```python
from build123d import *

# Parameters (mm, degrees)
ESQUISSE1_W        = 32
ESQUISSE1_H        = 3
BOSS_EXTRU_2_DEPTH = 2
ESQUISSE4_R        = 1.5
BOSS_EXTRU_3_DEPTH = 6
ESQUISSE5_R        = 1.9
BOSS_EXTRU_4_DEPTH = 1
CONG_13_R          = 1.5
CONG_14_R          = 1.5
CONG_16_R          = 1.5
CONG_17_R          = 1.5


with BuildPart() as part:
    # Esquisse1 → Boss.-Extru.2 (new body)
    with BuildSketch(Plane(origin=(-13.705479482, 0.648434545, 0), x_dir=(1, 0, 0), z_dir=(0, 0, 1))):
        with Locations((47.215800187, 12.683032093)):
            Rectangle(ESQUISSE1_W, ESQUISSE1_H)
    extrude(amount=BOSS_EXTRU_2_DEPTH)

    # Esquisse4 → Boss.-Extru.3 (add)
    with BuildSketch(Plane(origin=(-13.705479482, 4.052004393, 2), x_dir=(1, 0, 0), z_dir=(0, 0, 1))):
        with Locations(Location((32.71685212, 9.269475593, 0), (0, 0, 263.384796373))):
            Circle(ESQUISSE4_R)
        with Locations(Location((61.71685212, 9.250376763, 0), (0, 0, 258.698543871))):
            Circle(ESQUISSE4_R)
    extrude(amount=BOSS_EXTRU_3_DEPTH)

    # Esquisse5 → Boss.-Extru.4 (add)
    with BuildSketch(Plane(origin=(-13.705479482, 4.052004393, 8), x_dir=(1, 0, 0), z_dir=(0, 0, 1))):
        with Locations((32.71685212, 9.269475593)):
            Circle(ESQUISSE5_R)
        with Locations((61.71685212, 9.250376763)):
            Circle(ESQUISSE5_R)
    extrude(amount=BOSS_EXTRU_4_DEPTH)

    # Congé13
    # the kernel refuses this fillet: 1.5 mm, written as the material it takes off along each edge
    with BuildSketch(Plane(origin=(49.510320705, 14.831466639, -3.75), x_dir=(0, -1, 0), z_dir=(0, 0, 1)), Plane(origin=(49.510320705, 11.831466639, -3.75), x_dir=(-1, 0, 0), z_dir=(0, 0, 1))) as cong_13_piece_1:
        with BuildLine():
            CenterArc((CONG_13_R, -CONG_13_R), CONG_13_R, 90, 90)
            Line((0, -CONG_13_R), (0, 0))
            Line((0, 0), (CONG_13_R, 0))
        make_face()
    extrude(amount=5.75, mode=Mode.SUBTRACT)

    # Congé14
    # the kernel refuses this fillet: 1.5 mm, written as the material it takes off along each edge
    with BuildSketch(Plane(origin=(17.510320705, 11.831466639, -3.75), x_dir=(0, 1, 0), z_dir=(0, 0, 1))) as cong_14_piece_1:
        with BuildLine():
            CenterArc((CONG_14_R, -CONG_14_R), CONG_14_R, 90, 90)
            Line((0, -CONG_14_R), (0, 0))
            Line((0, 0), (CONG_14_R, 0))
        make_face()
    extrude(amount=5.75, mode=Mode.SUBTRACT)
    with BuildSketch(Plane(origin=(17.510320705, 14.831466639, -3.75), x_dir=(0, -1, 0), z_dir=(0, 0, 1))) as cong_14_piece_2:
        with BuildLine():
            CenterArc((CONG_14_R, CONG_14_R), CONG_14_R, 180, 90)
            Line((0, CONG_14_R), (0, 0))
            Line((0, 0), (CONG_14_R, 0))
        make_face()
    extrude(amount=9.5, mode=Mode.SUBTRACT)

    # Congé16
    # the kernel refuses this fillet: 1.5 mm, written as the material it takes off along each edge
    with BuildSketch(Plane(origin=(48.011372638, 13.302381156, 9), x_dir=(1, 0, 0), z_dir=(0, -1, 0))) as cong_16_piece_1:
        with BuildLine():
            CenterArc((0.485786438, -1.5), CONG_16_R, 19.471220634, 70.528779366)
            Line((0.485786438, 0), (0.485786438, 0.03))
            Line((0.485786438, 0.03), (1.9, 0.03))
            Line((1.9, 0.03), (1.93, 0))
            ThreePointArc((1.93, 0), (1.93, -0.5), (1.928284271, -0.99))
            Line((1.928284271, -0.99), (1.9, -1))
        make_face()
    revolve(axis=Axis((48.011372638, 13.302381156, 9), (0, 0, 1)), mode=Mode.SUBTRACT)

    # Congé17
    # the kernel refuses this fillet: 1.5 mm, written as the material it takes off along each edge
    with BuildSketch(Plane(origin=(19.011372638, 13.321479986, 9), x_dir=(1, 0, 0), z_dir=(0, -1, 0))) as cong_17_piece_1:
        with BuildLine():
            CenterArc((0.485786438, -1.5), CONG_17_R, 19.471220634, 70.528779366)
            Line((0.485786438, 0), (0.485786438, 0.03))
            Line((0.485786438, 0.03), (1.9, 0.03))
            Line((1.9, 0.03), (1.93, 0))
            ThreePointArc((1.93, 0), (1.93, -0.5), (1.928284271, -0.99))
            Line((1.928284271, -0.99), (1.9, -1))
        make_face()
    revolve(axis=Axis((19.011372638, 13.321479986, 9), (0, 0, 1)), mode=Mode.SUBTRACT)


solid = part.part
```
Input: part model. Units: mm. Frame: model coordinates. A direction names the side the tool comes from. Coordinates: 2 decimals unless noted, no trailing zeros. Write each loop counter-clockwise with the first axis right and the second up, starting at its lowest first coordinate (ties: lowest second). Pieces come first, ordered by that corner, then holes.
1) Section B-B on x = 34. Output: boundary loops of the cut face in (y, z), and give its area (3 significant figures).
2) Pin query (flat end, axial travel): pin 1 Ø0.6 at (x, z) = (34, 0.5) entering from +Y; pin 2 Ø1 at (y, z) = (14.5, 3.5) entering from +X; pin 3 Ø1.5 at (y, z) = (12, 3.5) entering from -X; pin 4 Ø4 at (x, z) = (24.5, 8) entering from +Y. Return the tip coordinate at first contact, or that it passes through.
3) Section A-A on z = 3.75. Output: boundary loops of the cut face in (x, y), and give its area (3 significant figures).
4) Material intervals for line 1 along Z through (x, y) = (25.5, 13.65); line 2 along X through (y, z) = (14.5, 6.25); line 3 along X through (y, z) = (14.6, 7.75), sorted ascending.
5) Mould query, pull axis X, two halves, no side actions, for faces 1 (the flat face through (33, 13, 0)), 2 (the flat face through (48, 15, 8)), 3 (the cylindrical face through (49.51, 13.3, 0.99)). Classes: pulls with the +X half, pulls with the -X half, needs draft (parallel to the pull), parting line crosses it, or undercut.
6) Set-up query: faces 4 (the flat face through (48, 13, 9)), 5 (the flat face through (20, 12, 8)), 6 (the cylindrical face through (17.51, 13.36, 0.99)). Return all of +Z, -Z, +X, -X, +Y, -Y with unobstructed straight access to the full face (end or side cutting, diameter ignored); none if empty.
Check result:
1. outline: (11.83, 0) - (14.83, 0) - (14.83, 2) - (11.83, 2) - close
1. area: 6.00 mm2
2. pin 1: stops at y = 14.83
2. pin 2: stops at x = 49.34
2. pin 3: stops at x = 17.62
2. pin 4: passes through
3. outline: circle Ø3 at (19.01, 13.32); circle Ø3 at (48.01, 13.3)
3. area: 14.1 mm2
4. line 1: z = 0 to 2
4. line 2: x = 18.08 to 19.94, 47.11 to 48.91
4. line 3: x = 18.23 to 19.8, 47.26 to 48.76
5. face 1: needs draft
5. face 2: undercut
5. face 3: pulls with the +X half
6. face 4: +Z, +X, -X, +Y, -Y
6. face 5: none
6. face 6: -Z, -X
